Build history of the part. All positions in model axes, mm. A direction names the side the tool comes from. Coordinates: 2 decimals unless noted, no trailing zeros. Order: outer loops, then holes, each group sorted by start corner. A loop starts at its lowest first (then second) coordinate and runs counter-clockwise, first axis right, second up. Notation, with made-up numbers: (49, 87.5) - (95, 87.5) arc R33 cw to (95, 122.5) - close; hole circle Ø2 at (-0.75, 34). An arc over 180 degrees is marked (long way). One line per item, written item: value.
from build123d import *

# Parameters (mm, degrees)
F0_W     = 94
F0_H     = 94
F0_W_2   = 90
F0_H_2   = 90.7552093267
F0_R     = 35
F1_DEPTH = 2
F2_DEPTH = 80
F3_R     = 3.5
F4_DEPTH = 100
F5_DEPTH = 150
F6_DEPTH = 94
F7_W     = 30
F7_H     = 5
F8_DEPTH = 100


with BuildPart() as f1:
    # F0 (on Top) → F1 (new body)
    with BuildSketch(Plane.XY):
        Rectangle(F0_W, F0_H)
        Rectangle(F0_W_2, F0_H_2, mode=Mode.SUBTRACT)
        Rectangle(F0_W_2, F0_H_2)
        Circle(F0_R, mode=Mode.SUBTRACT)
    extrude(amount=F1_DEPTH)

    # F0 (on Top) → F2 (join)
    with BuildSketch(Plane.XY):
        Rectangle(F0_W, F0_H)
        Rectangle(F0_W_2, F0_H_2, mode=Mode.SUBTRACT)
    extrude(amount=F2_DEPTH)

    # F3 (on face) → F4 (cut)
    with BuildSketch(Plane.XZ.offset(47)):
        with BuildLine():
            ThreePointArc((-12.5, 80), (0, 67.5), (12.5, 80))
            Line((12.5, 80), (-12.5, 80))
        make_face()
        with Locations((-34.9789150059, 17.0391555876)):
            Circle(F3_R)
    extrude(amount=-F4_DEPTH, mode=Mode.SUBTRACT)

    # F3 (on face) → F5 (cut)
    with BuildSketch(Plane.XZ.offset(47)):
        Polygon((-47, 37), (-14.5, 80), (-47, 80), align=None)
        Polygon((47, 80), (14.0333333333, 80), (47, 37), align=None)
    extrude(amount=-F5_DEPTH, mode=Mode.SUBTRACT)

    # F3 (on face) → F6 (join)
    with BuildSketch(Plane.XZ.offset(47)):
        Polygon((-47, 35), (-12.5, 80), (-14.5, 80), (-47, 37), align=None)
        Polygon((14.0333333333, 80), (12.5, 80), (47, 35), (47, 37), align=None)
    extrude(amount=-F6_DEPTH)

    # F7 (on face) → F8 (cut)
    with BuildSketch(Plane.YZ.offset(47)):
        with Locations((0, 66.8776729703)):
            Rectangle(F7_W, F7_H)
    extrude(amount=-F8_DEPTH, mode=Mode.SUBTRACT)


solid = f1.part
1. Probe line 1 along Y through (x, z) = (-16, 35); line 2 along X through (y, z) = (30, 27); line 3 along X through (y, z) = (-43, 46.5). List the from-to ranges inside material, lowest first.
Values found:
line 1: y = -47 to -45.38, 45.38 to 47
line 2: x = -47 to -45, 45 to 47
line 3: x = -39.82 to -38.18, 38.18 to 39.72
2. Band-saw the part on D-D, the plane x = -40. Give the cut face in (y, z), and give its area (3 significant figures).
Values found:
outline: (-47, 0) - (47, 0) - (47, 46.26) - (-47, 46.26) - close; hole (-45.38, 2) - (45.38, 2) - (45.38, 44.13) - (-45.38, 44.13) - close
area: 525 mm2
3. 3-axis set-ups, long thin cutter, end or side, ignore diameter. For faces 5 (the face through (-24, 15, 67)), 6 (the face through (45, -1, 20)), 7 (the face through (-32, 22, 0)): which of +Z, -Z, +X, -X, +Y, -Y reach the whole face in a straight line?
Values found:
face 5: +X, -X
face 6: none
face 7: -Z, +X, -X, +Y, -Y
4. Band-saw the part on C-C, the plane z = 23.5. Give the cut face in (x, y).
Values found:
outline: (-47, -47) - (47, -47) - (47, 47) - (-47, 47) - close; hole (-45, -45.38) - (45, -45.38) - (45, 45.38) - (-45, 45.38) - close
5. Flat gauge pins, fed straight in: P1, Ø1.2, axis at x = 21.5, y = -0.5, coming from the -Z side; P2, Ø4, axis at x = -34.98, z = 17.04, coming from the +Y side; P3, Ø1.5, axis at x = -25.5, y = 0.5, coming from the +Z side; P4, Ø6, axis at y = 33.5, z = 40.5, coming from the -X side. Where does each tip first touch, or does it go through?
Values found:
P1: stops at z = 69.38
P2: passes through
P3: stops at z = 64.38
P4: stops at x = -46.62
6. Two-plate mould, pull along Y, no slides. Class faces 1 (the face through (-24, -15, 67)), 2 (the face through (-1, 45.378, 32)), 3 (the face through (-0.275, -46.2, 67.503)), 4 (the face through (-1, 47, 31)): pulls with the +Y half, pulls with the -Y half, needs draft (parallel to the pull), parting line crosses it, or undercut.
Values found:
face 1: undercut
face 2: undercut
face 3: needs draft
face 4: pulls with the +Y half
7. Band-saw the part on A-A, the plane x = 0. Give the cut face in (y, z), and give its area (3 significant figures).
Values found:
outline: (-47, 0) - (-35, 0) - (-35, 2) - (-45.38, 2) - (-45.38, 67.5) - (-47, 67.5) - close; (35, 0) - (47, 0) - (47, 67.5) - (45.38, 67.5) - (45.38, 2) - (35, 2) - close
area: 261 mm2
8. Band-saw the part on B-B, the plane y = 0. Give the cut face in (x, z).
Values found:
outline: (-47, 0) - (-35, 0) - (-35, 2) - (-45, 2) - (-45, 37.61) - (-24.48, 64.38) - (-26.31, 64.38) - (-47, 37) - close; (-22.53, 69.38) - (-20.64, 69.38) - (-12.5, 80) - (-14.5, 80) - close; (12.5, 80) - (20.64, 69.38) - (22.18, 69.38) - (14.03, 80) - close; (24.48, 64.38) - (45, 37.61) - (45, 2) - (35, 2) - (35, 0) - (47, 0) - (47, 37) - (26.01, 64.38) - close
